```python
from build123d import *

# Parameters (mm, degrees)
SKETCH1_W                           = 35
SKETCH1_H                           = 65
BOSS_EXTRUDE1_DEPTH                 = 1
SKETCH2_W                           = 22.75
SKETCH2_H                           = 39
BOSS_EXTRUDE2_DEPTH                 = 13
HAI_LO_M3_TRUNG_TRU_TREO_DEPTH      = 40.134383859
HAI_LO_M3_TRUNG_TRU_TREO_DEPTH_BACK = 40.134383859
SKETCH4_R                           = 1.7


with BuildPart() as part:
    # Sketch1 → Boss-Extrude1 (new body)
    with BuildSketch(Plane.XY):
        Rectangle(SKETCH1_W, SKETCH1_H)
    extrude(amount=-BOSS_EXTRUDE1_DEPTH)

    # Sketch2 → Boss-Extrude2 (add)
    with BuildSketch(Plane.XY):
        Rectangle(SKETCH2_W, SKETCH2_H)
    extrude(amount=-BOSS_EXTRUDE2_DEPTH)

    # Sketch4 → Hai_lo_M3_trung_tru_treo (cut, two sides: drawn at the far end of the back side and taken through both)
    with BuildSketch(Plane.XY.offset(-HAI_LO_M3_TRUNG_TRU_TREO_DEPTH_BACK)):
        with Locations(Location((12.5, -30, 0), (0, 0, 180))):
            Circle(SKETCH4_R)
        with Locations(Location((12.5, 30, 0), (0, 0, 180))):
            Circle(SKETCH4_R)
    extrude(amount=HAI_LO_M3_TRUNG_TRU_TREO_DEPTH + HAI_LO_M3_TRUNG_TRU_TREO_DEPTH_BACK, mode=Mode.SUBTRACT)


solid = part.part
```
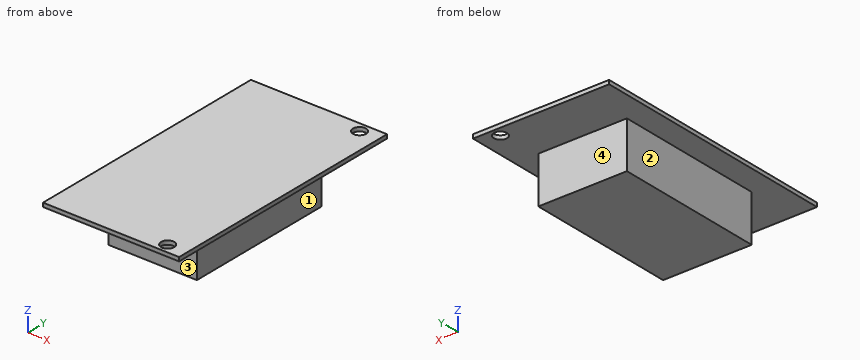
The model under review builds one solid part; all positions refer to its coordinate system, in mm. Face numbers are marked on the shaded views. A direction names the side the tool comes from. Give positions to 0.01 mm unless a question says otherwise; leave off trailing zeros. Write each loop counter-clockwise with the first axis right and the second up, starting at its lowest first coordinate (ties: lowest second). Pieces come first, ordered by that corner, then holes.
(1) Consider section D-D, the plane x = 1. Give the boundary of the cut face in (y, z), and give its area (3 significant figures).
(2) Tool access review of the marked faces 1, 2, 3 and 4: name each direction out of +Z, -Z, +X, -X, +Y, -Y from which nothing blocks a thin tool from reaching the whole face with its end or side.
(3) Consider section B-B, the plane x = 12.5. Give the boundary of the cut face in (y, z).
(4) Consider section C-C, the plane y = 17. Give the boundary of the cut face in (x, z) (3 decimals), and give its area (3 significant figures).
(5) For P1, Ø10, axis at x = -1.5, y = 9.5, coming from the +Z side; P2, Ø3.5, axis at y = -8, z = -8, coming from the +X side (3 decimals); P3, Ø3, axis at x = 12.5, y = -30, coming from the +Z side; P4, Ø1.5, axis at x = 5.5, z = -9, coming from the +Y side, all flat-tipped, find the tip position at first contact; note any pin that passes through.
(6) Consider section A-A, the plane y = -30. Give the boundary of the cut face in (x, z), and give its area (3 significant figures).
(7) To check wall thickness, follow L1, parallel to Y at x = 12.5, z = -0.7; L2, parallel to Z at x = 7.5, y = 23.5; L3, parallel to X at y = 8, z = -11.25 (3 decimals). State the ranges of each line that lie inside material, in increasing order.
Returned:
1. outline: (-32.5, -1) - (-19.5, -1) - (-19.5, -13) - (19.5, -13) - (19.5, -1) - (32.5, -1) - (32.5, 0) - (-32.5, 0) - close
1. area: 533 mm2
2. face 1: -Z, +X, +Y, -Y
2. face 2: -Z, -X, +Y, -Y
2. face 3: -Z, +X, -X, -Y
2. face 4: -Z, +X, -X, +Y
3. outline: (-32.5, -1) - (-31.7, -1) - (-31.7, 0) - (-32.5, 0) - close; (-28.3, -1) - (28.3, -1) - (28.3, 0) - (-28.3, 0) - close; (31.7, -1) - (32.5, -1) - (32.5, 0) - (31.7, 0) - close
4. outline: (-17.5, -1) - (-11.375, -1) - (-11.375, -13) - (11.375, -13) - (11.375, -1) - (17.5, -1) - (17.5, 0) - (-17.5, 0) - close
4. area: 308 mm2
5. P1: stops at z = 0
5. P2: stops at x = 11.375
5. P3: passes through
5. P4: stops at y = 19.5
6. outline: (-17.5, -1) - (10.8, -1) - (10.8, 0) - (-17.5, 0) - close; (14.2, -1) - (17.5, -1) - (17.5, 0) - (14.2, 0) - close
6. area: 31.6 mm2
7. L1: y = -32.5 to -31.7, -28.3 to 28.3, 31.7 to 32.5
7. L2: z = -1 to 0
7. L3: x = -11.375 to 11.375
